Design review of the part built by this model. Coordinates are the model's own, in mm. Face numbers are marked on the shaded views. A direction names the side the tool comes from. Round coordinates to 2 decimals unless told otherwise and drop trailing zeros. Order: outer loops, then holes, each group sorted by start corner. A loop starts at its lowest first (then second) coordinate and runs counter-clockwise, first axis right, second up.
Autodesk Inventor part; units mm, degrees
ref_plane "YZ Plane" through (0, 0, 0) normal (1, 0, 0) x (0, 1, 0)
ref_plane "XZ Plane" through (0, 0, 0) normal (0, 1, 0) x (-1, 0, 0)
ref_plane "XY Plane" through (0, 0, 0) normal (0, 0, 1) x (1, 0, 0)
sketch "Sketch1" plane through (0, 0, 0) normal (0, 1, 0) x (-1, 0, 0)
  line L0 (0, 0) -> (28, 0)
  line L1 (28, 0) -> (28, -28)
  line L2 (28, -28) -> (0, -28)
  line L3 (0, -28) -> (0, 0)
  line L4 (24.125, -3.875) -> (3.875, -3.875)
  line L5 (3.875, -3.875) -> (3.875, -24.125)
  line L6 (3.875, -24.125) -> (24.125, -24.125)
  line L7 (24.125, -24.125) -> (24.125, -3.875)
  line L8 (24.125, -3.875) -> (3.875, -24.125) construction
  line L9 (3.875, -3.875) -> (24.125, -24.125) construction
  line L10 (0, 0) -> (28, -28) construction
  line L11 (28, 0) -> (0, -28) construction
  point P0 (14, -14)
  dimension "d0" = 28
  dimension "d1" = 28
  dimension "d2" = 20.25
  dimension "d3" = 20.25
extrude "Extrusion1" add sketch "Sketch1" along normal blind 15
fillet "Fillet1" radius 0.6 8 edges at (-14, 0, -3.875) (-24.125, 0, -14) (-14, 0, -24.125) (-3.875, 0, -14) (-14, 0, 0) (-28, 0, -14) (-14, 0, -28) (0, 0, -14)
sketch "Sketch2" plane through (-28, 15, -28) normal (-1, 0, 0) x (0, 0, 1)
  circle A0 centre (14, -8.7403) radius 1.75
  point P0 (28, -15)
  dimension "d7" = 3.5
extrude "Extrusion2" cut sketch "Sketch2" against normal blind 10
sketch "Sketch3" plane through (0, 15, 0) normal (1, 0, 0) x (0, 0, -1)
  circle A0 centre (14, -8.7403) radius 1.75
  circle A1 centre (14, -8.7403) radius 1.75
  point P0 (0, -15)
  dimension "d10" = 3.5
extrude "Extrusion3" cut sketch "Sketch3" against normal blind 10
fillet "Fillet2" radius 0.5 2 edges at (-3.875, 6.2597, -12.25) (-24.125, 6.2597, -15.75)
properties part number "TestSujetaPerfil"
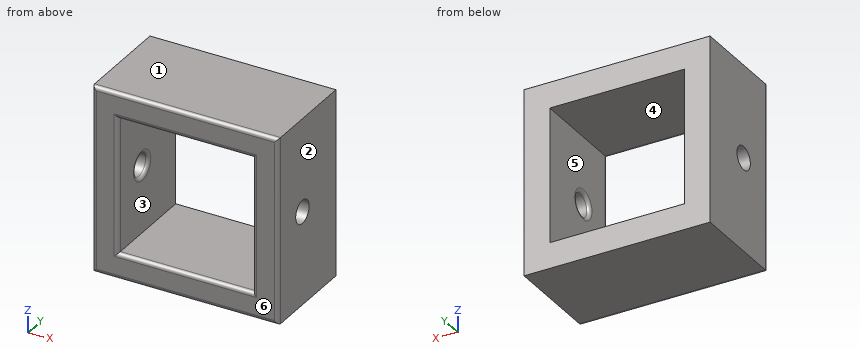
1) For the marked faces 5 and 6, list the 3-axis set-ups (+Z, -Z, +X, -X, +Y, -Y) from which the entire face can be reached by the end or side of a thin tool; tool diameter is ignored.
Results:
face 5: +Y, -Y
face 6: +Z, -Z, +X, -X, -Y
2) Take a section at A-A on x = -8.5. Give the boundary of the cut face in (y, z) (3 decimals), plus the area to 3 significant figures.
Results:
outline: (0, -27.4) arc R0.6 ccw to (0.6, -28) - (15, -28) - (15, -24.125) - (0.6, -24.125) arc R0.6 ccw to (0, -24.725) - close; (0, -3.275) arc R0.6 ccw to (0.6, -3.875) - (15, -3.875) - (15, 0) - (0.6, 0) arc R0.6 ccw to (0, -0.6) - close
area: 116 mm2
3) Take a section at C-C on y = 13. Give the boundary of the cut face in (x, z) (3 decimals), plus the area to 3 significant figures.
Results:
outline: (-28, -28) - (0, -28) - (0, 0) - (-28, 0) - close; hole (-24.125, -24.125) - (-3.875, -24.125) - (-3.875, -3.875) - (-24.125, -3.875) - close
area: 374 mm2
4) To check wall thickness, follow line 1 along Z through (x, y) = (-7.5, 6.5) (3 decimals); line 2 along Y through (x, z) = (-2.35, -14). State the ranges of each line that lie inside material, in increasing order.
Results:
line 1: z = -28 to -24.125, -3.875 to 0
line 2: y = 0 to 4.51, 8.01 to 15
5) Take a section at D-D on z = -14. Give the boundary of the cut face in (x, y) (3 decimals).
Results:
outline: (-28, 0.6) arc R0.6 ccw to (-27.4, 0) - (-24.725, 0) arc R0.6 ccw to (-24.125, 0.6) - (-24.125, 4.01) arc R0.5 ccw to (-24.625, 4.51) - (-28, 4.51) - close; (-28, 8.01) - (-24.625, 8.01) arc R0.5 ccw to (-24.125, 8.51) - (-24.125, 15) - (-28, 15) - close; (-3.875, 0.6) arc R0.6 ccw to (-3.275, 0) - (-0.6, 0) arc R0.6 ccw to (0, 0.6) - (0, 4.51) - (-3.375, 4.51) arc R0.5 ccw to (-3.875, 4.01) - close; (-3.875, 8.51) arc R0.5 ccw to (-3.375, 8.01) - (0, 8.01) - (0, 15) - (-3.875, 15) - close
6) Clearance check with a flat-ended pin moving along its axis: P1, Ø3, axis at y = 6.26, z = -14, coming from the +X side. State where the tip first meets the part, or that it passes through.
Results:
P1: passes through
7) The part is to be moulded in two halves that separate along X. For the marked faces 1, 2, 3 and 4, say which applies: released by +X, released by -X, zero draft, split by the parting line, or undercut.
Results:
face 1: zero draft
face 2: released by +X
face 3: undercut
face 4: undercut
8) Take a section at B-B on z = -5.5. Give the boundary of the cut face in (x, y) (3 decimals).
Results:
outline: (-28, 0.6) arc R0.6 ccw to (-27.4, 0) - (-24.725, 0) arc R0.6 ccw to (-24.125, 0.6) - (-24.125, 15) - (-28, 15) - close; (-3.875, 0.6) arc R0.6 ccw to (-3.275, 0) - (-0.6, 0) arc R0.6 ccw to (0, 0.6) - (0, 15) - (-3.875, 15) - close
